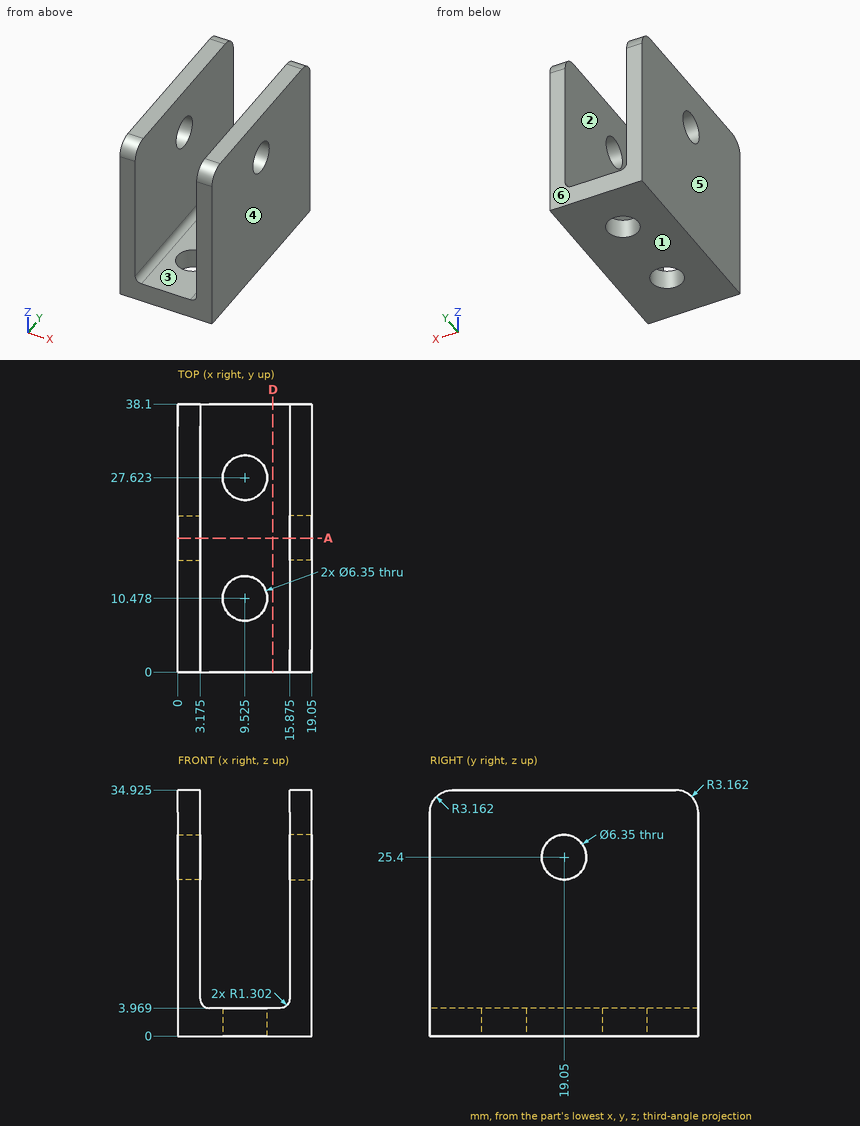
Here's the drawing with two shaded views (mm, measured from the low corner). I have some questions. A direction names the side the tool comes from. Coordinates: 2 decimals unless noted, no trailing zeros. Write each loop counter-clockwise with the first axis right and the second up, starting at its lowest first coordinate (ties: lowest second). Pieces come first, ordered by that corner, then holes. Notation, with made-up numbers: (-27, -22.75) -> (-6, -22.75) arc R25 cw to (-6, 2.25) -> close; hole circle Ø8 at (-6, 33.25). An arc over 180 degrees is marked (long way). Write item = value, one per line. Start each with the question number.
(1) I want a section at A-A (y = 19.05). Give the number of separate pieces and of enclosed holes in the cut face.
(2) Which directions (+Z, -Z, +X, -X, +Y, -Y) give clear straight access to the entire face, cutting with the end or side of a thin tool? Please do the marked faces 1 and 2.
(3) Will this pin go through, and if not, where does the flat tip stop? pin 1 (8 mm diameter, centred on x = 8.5, y = 18.5, fed in from +Z).
(4) I need wall thicknesses on line 1 (Y direction, x = 7.75, z = 2) (1 decimal); line 2 (Y direction, x = 18.3, z = 25.4) (1 decimal); line 3 (Y direction, x = 7.5, z = 3) (1 decimal). Which ranges of each line are inside material? Lowest first, please. Write a range as [from, to].
(5) I want a section at D-D (x = 13.5). Please give me the cut outline in (y, z), plus the area to 3 significant figures.
(6) We'd pull the mould along X, two halves only. Please class the marked faces 3, 4, 5 and 6: released by +X, released by -X, zero draft, split by the parting line, or undercut.
Result set:
q1.separate_pieces = 3
q1.enclosed_holes = 0
q2.face_1 = -Z, +X, -X, +Y, -Y
q2.face_2 = +Z, +Y, -Y
q3.pin_1 = 3.97
q4.line_1 = [0, 7.8], [13.1, 25], [30.3, 38.1]
q4.line_2 = [0, 15.9], [22.2, 38.1]
q4.line_3 = [0, 8], [12.9, 25.2], [30.1, 38.1]
q5.outline = (0, 0) -> (38.1, 0) -> (38.1, 3.97) -> (0, 3.97) -> close
q5.area = 151 mm2
q6.face_3 = undercut
q6.face_4 = released by +X
q6.face_5 = released by -X
q6.face_6 = zero draft
